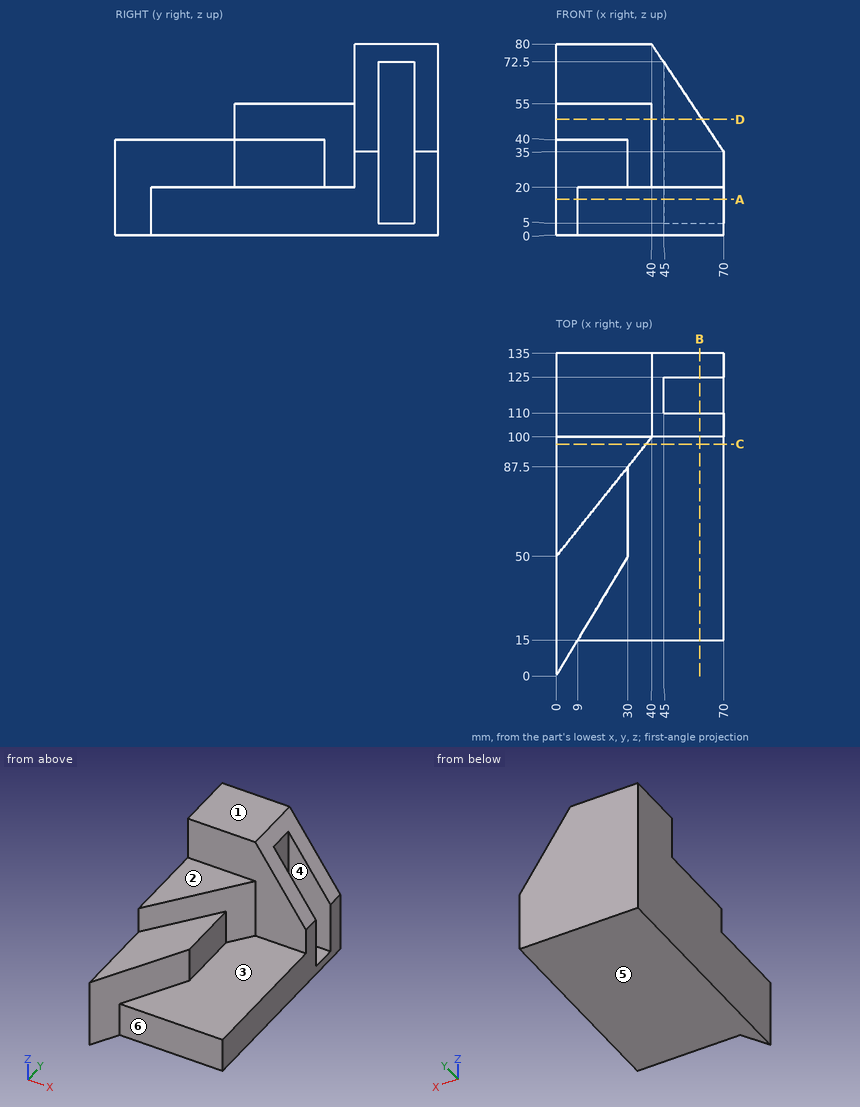
Part print with two shaded views. Sizes in mm from the minimum x, y, z corner. A direction names the side the tool comes from. Round coordinates to 2 decimals unless told otherwise and drop trailing zeros. Loops run counter-clockwise (first coordinate to the right, second up) from the corner with the lowest first, then second, coordinate; pieces in that order, holes last. Notation, with made-up numbers: (-4, 59.25) - (44, 59.25) arc R18 ccw to (44, 80.25) - close; hole circle Ø8 at (30, 84). An arc over 180 degrees is marked (long way). Answer as a JSON object with one key per item and string values.
Item 1: Tool access for the marked faces 1, 2 and 3: list every direction of +Z, -Z, +X, -X, +Y, -Y with a clear straight run to the whole face (end or side of a thin tool).
Output:
{"face 1": "+Z, +X, -X, +Y, -Y", "face 2": "+Z, +X, -X, -Y", "face 3": "+Z, +X, -Y"}
Item 2: Band-saw the part on C-C on y = 97. List the corners of the cut face in (x, z), plus the area to 3 significant figures.
Output:
{"outline": "(0, 0) - (70, 0) - (70, 20) - (37.6, 20) - (37.6, 55) - (0, 55) - close", "area": "2,720 mm2"}
Item 3: Band-saw the part on B-B on x = 60. List the corners of the cut face in (y, z), plus the area to 4 significant figures.
Output:
{"outline": "(15, 0) - (135, 0) - (135, 50) - (125, 50) - (125, 5) - (110, 5) - (110, 50) - (100, 50) - (100, 20) - (15, 20) - close", "area": "2,775 mm2"}
Item 4: Pin check, flat tips, straight feed: pin 1 (6 mm diameter, centred on y = 76.5, z = 30.5, fed in from +X); pin 2 (22 mm diameter, centred on x = 27, z = 10.5, fed in from -Y); pin 3 (15 mm diameter, centred on x = 22, y = 37, fed in from +Z). Stop position of each tip, or through.
Output:
{"pin 1": "x = 30", "pin 2": "y = 15", "pin 3": "z = 40"}
Item 5: Wall check: L1, parallel to Y at x = 60, z = 16; L2, parallel to Y at x = 52.5, z = 34; L3, parallel to Y at x = 14, z = 14. Give the ranges that are in metal, low to high.
Output:
{"L1": "15 to 110, 125 to 135", "L2": "100 to 110, 125 to 135", "L3": "15 to 135"}
Item 6: Band-saw the part on A-A on z = 15. List the corners of the cut face in (x, y).
Output:
{"outline": "(0, 0) - (9, 15) - (70, 15) - (70, 110) - (45, 110) - (45, 125) - (70, 125) - (70, 135) - (0, 135) - close"}
Item 7: Pull direction Y, two halves, no side cores. Call the marked faces 4, 5 and 6: pulls with the +Y half, pulls with the -Y half, needs draft (parallel to the pull), parting line crosses it, or undercut.
Output:
{"face 4": "undercut", "face 5": "needs draft", "face 6": "pulls with the -Y half"}
Item 8: Band-saw the part on D-D on z = 48.5. List the corners of the cut face in (x, y), plus the area to 4 significant figures.
Output:
{"outline": "(0, 50) - (40, 100) - (61, 100) - (61, 110) - (45, 110) - (45, 125) - (61, 125) - (61, 135) - (0, 135) - close", "area": "2,895 mm2"}
